Work out the finished part from the listing and answer in its coordinate system (mm). Round coordinates to 2 decimals unless told otherwise and drop trailing zeros. Order: outer loops, then holes, each group sorted by start corner. A loop starts at its lowest first (then second) coordinate and runs counter-clockwise, first axis right, second up. Notation, with made-up numbers: (89, -27) - (103, -27) arc R23 ccw to (103, 7) - close; hole circle Ø6 at (87, 86). An arc over 180 degrees is marked (long way). Answer in a Markdown table with one row per item.
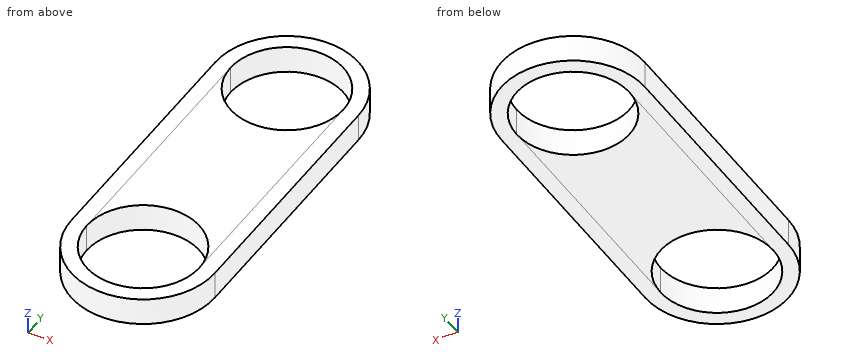
from build123d import *
from build123d.topology import SkipClean

# Parameters (mm, degrees)
BOSS_EXTRUDE1_DEPTH = 5


with BuildPart() as part:
    # Sketch1 → Boss-Extrude1 (new body)
    # profile 1 of 2: a face of its own
    with SkipClean():  # the faces are left unmerged after this step: merging them gives an invalid solid
        with BuildSketch(Plane.XY):
            with BuildLine():
                Line((-13, 0), (-13, -45))
                ThreePointArc((-13, -45), (0, -58), (13, -45))
                Line((13, -45), (13, 0))
                ThreePointArc((13, 0), (0, 13), (-13, 0))
            make_face()
            with BuildLine():
                ThreePointArc((-10.25, -45), (0, -55.25), (10.25, -45))
                Line((10.25, -45), (10.25, 0))
                ThreePointArc((10.25, 0), (0, 10.25), (-10.25, 0))
                Line((-10.25, 0), (-10.25, -45))
            make_face(mode=Mode.SUBTRACT)
        # profile 2 of 2: a face of its own
        with BuildSketch(Plane.XY):
            with BuildLine():
                Line((10.25, -45), (10.25, 0))
                ThreePointArc((10.25, 0), (0, -10.25), (-10.25, 0))
                Line((-10.25, 0), (-10.25, -45))
                ThreePointArc((-10.25, -45), (0, -34.75), (10.25, -45))
            make_face()
        extrude(amount=BOSS_EXTRUDE1_DEPTH)
    add(part.part.scale(1), mode=Mode.REPLACE)  # the faces are merged on a copy


solid = part.part
1) Find section C-C, the plane y = 4. Give the vertices of the cut face in (x, z).
Filled in:
| item | result |
|---|---|
| outline | (-12.37, 0) - (-9.44, 0) - (-9.44, 5) - (-12.37, 5) - close; (9.44, 0) - (12.37, 0) - (12.37, 5) - (9.44, 5) - close |
2) Find section D-D, the plane x = -5. Give the vertices of the cut face in (y, z), then the cut area to 3 significant figures.
Filled in:
| item | result |
|---|---|
| outline | (-57, 0) - (-53.95, 0) - (-53.95, 5) - (-57, 5) - close; (-36.05, 0) - (-8.95, 0) - (-8.95, 5) - (-36.05, 5) - close; (8.95, 0) - (12, 0) - (12, 5) - (8.95, 5) - close |
| area | 166 mm^2 |
3) This flat-tipped pin is pushed along its axis until it touches: pin 1 (2 mm diameter, centred on x = -0.5, z = 3, fed in from +Y). Where does it stop, or does it pass through?
Filled in:
| item | result |
|---|---|
| pin 1 | stops at y = 13 |
4) Find the intervals of material crossed by probe 1 along Y at (x, z) = (0.5, 0.9); probe 2 along Y at (x, z) = (-9.25, 2.85); probe 3 along X at (y, z) = (2, 3), in increasing order. Write a range as from..to.
Filled in:
| item | result |
|---|---|
| probe 1 | y = -57.99..-55.24, -34.76..-10.24, 10.24..12.99 |
| probe 2 | y = -54.13..-49.42, -40.58..-4.42, 4.42..9.13 |
| probe 3 | x = -12.85..-10.05, 10.05..12.85 |
5) Find section B-B, the plane z = 2.2. Give the vertices of the cut face in (x, y).
Filled in:
| item | result |
|---|---|
| outline | (-13, -45) arc R13 ccw to (13, -45) - (13, 0) arc R13 ccw to (-13, 0) - close; hole circle Ø20.5 at (0, -45); hole circle Ø20.5 at (0, 0) |
6) Find section A-A, the plane x = 0. Give the vertices of the cut face in (y, z).
Filled in:
| item | result |
|---|---|
| outline | (-58, 0) - (-55.25, 0) - (-55.25, 5) - (-58, 5) - close; (-34.75, 0) - (-10.25, 0) - (-10.25, 5) - (-34.75, 5) - close; (10.25, 0) - (13, 0) - (13, 5) - (10.25, 5) - close |
